Solid Edge part; units mm, degrees
sketch "Sketch1" plane through (0, 0, 0) normal (0, 0, 1) x (1, 0, 0)
  line L0 (-46.5, -60) -> (46.5, -60)
  line L1 (46.5, -60) -> (46.5, 60)
  line L2 (46.5, 60) -> (-46.5, 60)
  line L3 (-46.5, 60) -> (-46.5, -60)
extrude "Protrusion1" add sketch "Sketch1" along normal blind 2
sketch "Sketch2" plane through (0, 0, 2) normal (0, 0, 1) x (1, 0, 0)
  arc A0 (-16.5, 5) -> (-16.5, -5) centre (-16.5, 0) cw
  line L0 (-16.5, 5) -> (-46.5, 5)
  line L1 (-46.5, 5) -> (-46.5, -5)
  line L2 (-46.5, -5) -> (-16.5, -5)
  line L3 (-16.5, 8.5) -> (16.5, 8.5)
  line L4 (16.5, 8.5) -> (16.5, 41.5)
  line L5 (16.5, 41.5) -> (-16.5, 41.5)
  line L6 (-16.5, 41.5) -> (-16.5, 8.5)
  line L7 (13, -12) -> (-13, -12)
  line L8 (-13, -12) -> (-13, -38)
  line L9 (-13, -38) -> (13, -38)
  line L10 (13, -38) -> (13, -12)
extrude "Cutout1" cut sketch "Sketch2" against normal up to next
Work out the finished part from the listing and answer in its coordinate system (mm). Give positions to 0.01 mm unless a question says otherwise; leave off trailing zeros. Order: outer loops, then holes, each group sorted by start corner. A loop starts at its lowest first (then second) coordinate and runs counter-clockwise, first axis right, second up. Notation, with made-up numbers: (-7, -10) - (49, -10) arc R22 ccw to (49, 10) - close; hole circle Ø5 at (-25, 6.25). An arc over 180 degrees is marked (long way). Answer as CSV lines item,"result". Start each with the question number.
Q1. The part is cut by section A-A (y = -29.5). Write down the section's boundary in (x, z).
Q2. The part is cut by section D-D (y = -3). Write down the section's boundary in (x, z).
Q3. The part is cut by section B-B (x = -38.5). Write down the section's boundary in (y, z), then the cut area to 3 significant figures.
Q4. The part is cut by section C-C (z = 1). Write down the section's boundary in (x, y).
Q5. Find the intervals of material crossed by L1, parallel to Y at x = -5.5, z = 1.1; L2, parallel to X at y = 18.5, z = 1.7; L3, parallel to Y at x = -31.5, z = 0.85, in increasing order. Write a range as [from, to].
Check result:
1,outline,"(-46.5, 0) - (-13, 0) - (-13, 2) - (-46.5, 2) - close; (13, 0) - (46.5, 0) - (46.5, 2) - (13, 2) - close"
2,outline,"(-12.5, 0) - (46.5, 0) - (46.5, 2) - (-12.5, 2) - close"
3,outline,"(-60, 0) - (-5, 0) - (-5, 2) - (-60, 2) - close; (5, 0) - (60, 0) - (60, 2) - (5, 2) - close"
3,area,"220 mm²"
4,outline,"(-46.5, -60) - (46.5, -60) - (46.5, 60) - (-46.5, 60) - (-46.5, 5) - (-16.5, 5) arc R5 cw to (-16.5, -5) - (-46.5, -5) - close; hole (-16.5, 8.5) - (16.5, 8.5) - (16.5, 41.5) - (-16.5, 41.5) - close; hole (-13, -38) - (13, -38) - (13, -12) - (-13, -12) - close"
5,L1,"y = [-60, -38], [-12, 8.5], [41.5, 60]"
5,L2,"x = [-46.5, -16.5], [16.5, 46.5]"
5,L3,"y = [-60, -5], [5, 60]"
